```python
from build123d import *

# Parameters (mm, degrees)
SKETCH1_R           = 42.5
SKETCH1_R_2         = 20
BOSS_EXTRUDE1_DEPTH = 30
SKETCH2_R           = 32.5
SKETCH2_R_2         = 20
BOSS_EXTRUDE2_DEPTH = 780
SKETCH3_R           = 32.5
BOSS_EXTRUDE3_DEPTH = 5
SKETCH4_R           = 15
BOSS_EXTRUDE4_DEPTH = 65
SKETCH5_R           = 30
SKETCH5_R_2         = 15
BOSS_EXTRUDE5_DEPTH = 40
FILLET1_R           = 5


with BuildPart() as part:
    # Sketch1 → Boss-Extrude1 (new body)
    with BuildSketch(Plane.XY):
        Circle(SKETCH1_R)
        Circle(SKETCH1_R_2, mode=Mode.SUBTRACT)
    extrude(amount=-BOSS_EXTRUDE1_DEPTH)

    # Sketch2 → Boss-Extrude2 (add)
    with BuildSketch(Plane(origin=(0, 0, -30), x_dir=(-1, 0, 0), z_dir=(0, 0, -1))):
        with Locations(Location((0, 0, 0), (0, 0, 180))):
            Circle(SKETCH2_R)
        with Locations(Location((0, 0, 0), (0, 0, 180))):
            Circle(SKETCH2_R_2, mode=Mode.SUBTRACT)
    extrude(amount=BOSS_EXTRUDE2_DEPTH)

    # Sketch3 → Boss-Extrude3 (add)
    with BuildSketch(Plane(origin=(0, 0, -810), x_dir=(-1, 0, 0), z_dir=(0, 0, -1))):
        with Locations(Location((0, 0, 0), (0, 0, 180))):
            Circle(SKETCH3_R)
    extrude(amount=BOSS_EXTRUDE3_DEPTH)

    # Sketch4 → Boss-Extrude4 (add)
    with BuildSketch(Plane(origin=(0, 0, -815), x_dir=(-1, 0, 0), z_dir=(0, 0, -1))):
        Circle(SKETCH4_R)
    extrude(amount=BOSS_EXTRUDE4_DEPTH)

    # Sketch5 → Boss-Extrude5 (add, symmetric)
    with BuildSketch(Plane(origin=(0, 0, 0), x_dir=(0, 0, -1), z_dir=(1, 0, 0))):
        with Locations((905, 0)):
            Circle(SKETCH5_R)
        with Locations((905, 0)):
            Circle(SKETCH5_R_2, mode=Mode.SUBTRACT)
    extrude(amount=BOSS_EXTRUDE5_DEPTH, both=True)

    # Fillet1
    fillet1_edges = [part.edges().sort_by_distance(p)[0] for p in [
        (-32.5, 0, -30),
        (-32.5, 0, -815),
        (15, 0, -815),
        (-42.5, 0, -30),
    ]]
    fillet(fillet1_edges, radius=FILLET1_R - 0.0001)  # a hair under: the kernel refuses the full size


solid = part.part
```
Check sheet for the modelled part. Datum: model origin and axes. Units: mm. A direction names the side the tool comes from. Coordinates: 2 decimals unless noted, no trailing zeros. Loops run counter-clockwise (first coordinate to the right, second up) from the corner with the lowest first, then second, coordinate; pieces in that order, holes last.
1) Access from +Z, -Z, +X, -X, +Y, -Y to the whole of each face (thin tool, end or side, straight path). Record for faces 5 (the face through (-0.56, -5.745, -918.856)), 6 (the face through (1.9, 20.2, -815)), 7 (the face through (40, 14, -911)).
2) Release check for a two-part mould opening along X. For faces 1 (the face through (8.8, -18.3, 0)), 2 (the face through (-40, 14, -911)), 3 (the face through (-33.727, -25.861, -12.325)), 4 (the face through (0, 0, -810)) record: released by +X, released by -X, zero draft, split by the parting line, or undercut.
3) Gauge pin test, flat ends, axial feed: pin 1 (24 mm diameter, centred on x = 0, y = 0, fed in from +Z); pin 2 (1.5 mm diameter, centred on y = 20.5, z = -461.5, fed in from -X); pin 3 (1 mm diameter, centred on x = -14.5, z = -147.5, fed in from -Y). Record the tip position at first contact, or that the pin passes through.
4) Sectioned sample at D-D (z = -60). Record the boundary of the cut face in (x, y).
5) Material ranges on probe 1 along Z at (x, y) = (-16, 7.5); probe 2 along Z at (x, y) = (27, 9); probe 3 along Z at (x, y) = (-2, -2), recorded low to high.
6) Sectioned sample at B-B (z = -905). Record the boundary of the cut face in (x, y), and give its area (3 significant figures).
Check sheet entries:
1. face 5: +X, -X
1. face 6: none
1. face 7: -Z, +X, +Y, -Y
2. face 1: zero draft
2. face 2: released by -X
2. face 3: split by the parting line
2. face 4: undercut
3. pin 1: stops at z = -810
3. pin 2: stops at x = -25.81
3. pin 3: stops at y = -29.33
4. outline: circle Ø65 at (0, 0); hole circle Ø40 at (0, 0)
5. probe 1: z = -934.05 to -917.99, -892.01 to -875.95, -815.58 to -810
5. probe 2: z = -933.62 to -917, -893 to -876.38, -814.91 to 0
5. probe 3: z = -934.93 to -919.87, -890.13 to -810
6. outline: (-40, -30) - (40, -30) - (40, -15) - (-40, -15) - close; (-40, 15) - (40, 15) - (40, 30) - (-40, 30) - close
6. area: 2,400 mm2
